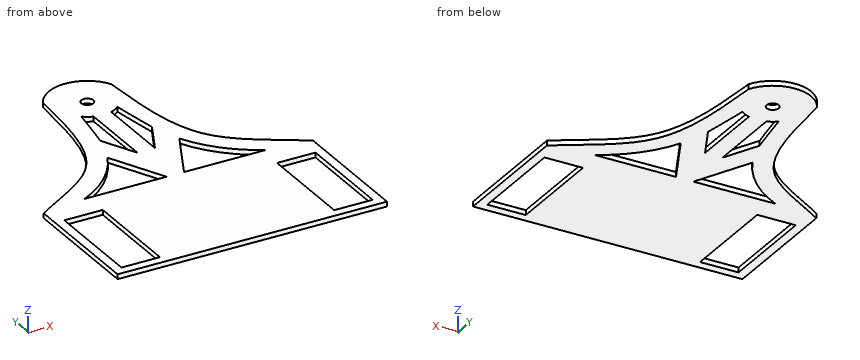
```python
from build123d import *

# Parameters (mm, degrees)
F0_R     = 4
F0_W     = 177.8
F0_H     = 85.24
F0_W_2   = 25.4
F0_H_2   = 66.04
F1_DEPTH = 3.175


with BuildPart() as f1:
    # F0 (on Top) → F1 (new body)
    with BuildSketch(Plane.XY):
        with BuildLine():
            add(Edge.make_bspline(
                [(22.5202294805, 113.3473088044), (24.6785630933, 84.2312430336), (27.5522275569, 27.268327843), (69.7704020362, 9.5247320193), (88.8999999985, -3.66)],
                knots=[0, 0, 0, 0, 0.529467504, 1, 1, 1, 1], degree=3))
            ThreePointArc((22.5202294805, 113.3473088043), (1e-10, 127), (-22.5202294805, 113.3473088044))
            add(Edge.make_bspline(
                [(-22.5202294805, 113.3473088044), (-24.6785630933, 84.2312430336), (-27.5522275569, 27.268327843), (-69.7704020362, 9.5247320193), (-88.8999999985, -3.66)],
                knots=[0, 0, 0, 0, 0.529467504, 1, 1, 1, 1], degree=3))
            Line((-88.8999999985, -3.66), (88.9000000015, -3.66))
        make_face()
        with BuildLine():
            ThreePointArc((-59.8212145269, 0), (-38.7136496278, 15.4052324982), (-23.6512337148, 36.7587828155))
            Line((-23.6512337148, 36.7587828155), (-5.7622946509, 0))
            Line((-5.7622946509, 0), (-59.8212145269, 0))
        make_face(mode=Mode.SUBTRACT)
        with BuildLine():
            Line((5.7622946509, 0), (23.6512337148, 36.7587828155))
            ThreePointArc((23.6512337148, 36.7587828155), (38.7136496278, 15.4052324982), (59.8212145269, 0))
            Line((59.8212145269, 0), (5.7622946509, 0))
        make_face(mode=Mode.SUBTRACT)
        with BuildLine():
            Line((-5.7622946509, 33.5634882355), (-17.0102279312, 56.676113031))
            ThreePointArc((-17.0102279312, 56.676113031), (-14.345117084, 72.11901875), (-11.9453535958, 87.6053768783))
            ThreePointArc((-11.9453535958, 87.6053768783), (-9.0231108807, 85.5649004094), (-5.7622946509, 84.1261077832))
            Line((-5.7622946509, 84.1261077832), (-5.7622946509, 33.5634882355))
        make_face(mode=Mode.SUBTRACT)
        with Locations((0, 101.6)):
            Circle(F0_R, mode=Mode.SUBTRACT)
        with BuildLine():
            Line((5.7622946509, 33.5634882355), (5.7622946509, 84.1261077832))
            ThreePointArc((5.7622946509, 84.1261077832), (9.0231108807, 85.5649004094), (11.9453535958, 87.6053768783))
            ThreePointArc((11.9453535958, 87.6053768783), (14.345117084, 72.11901875), (17.0102279312, 56.676113031))
            Line((17.0102279312, 56.676113031), (5.7622946509, 33.5634882355))
        make_face(mode=Mode.SUBTRACT)
        with Locations((1.5e-09, -46.28)):
            Rectangle(F0_W, F0_H)
        with Locations((-70.1999999985, -49.88)):
            Rectangle(F0_W_2, F0_H_2, mode=Mode.SUBTRACT)
        with Locations((70.1999999985, -49.88)):
            Rectangle(F0_W_2, F0_H_2, mode=Mode.SUBTRACT)
    extrude(amount=F1_DEPTH)


solid = f1.part
```
Source: CAD feature listing. Evaluate the final solid. Frame: model axes, mm. Coordinates: 2 decimals unless noted, no trailing zeros. Write each loop counter-clockwise with the first axis right and the second up, starting at its lowest first coordinate (ties: lowest second). Pieces come first, ordered by that corner, then holes. Notation, with made-up numbers: M 19,61 L 36,61 A33 ccw 36,97 Z; hole C -9,6.5 d3. An arc over 180 degrees is marked long. Answer as a JSON object with one key per item and string values.
1. Contact query for flat-ended pins moving along their axis: P1, Ø1, axis at x = -41.5, z = 2.5, coming from the +Y side; P2, Ø6.5, axis at x = 0, y = 101.6, coming from the -Z side; P3, Ø1, axis at x = 68.5, z = 2.5, coming from the +Y side. Output: stop coordinate, or through.
Evaluation:
{"P1": "y = 31.74", "P2": "through", "P3": "y = 9.58"}
2. Cut plane D-D on x = 20. Output: boundary loops of the cut face in (y, z) (3 decimals).
Evaluation:
{"outline": "M -88.9,0 L 0,0 L 0,3.175 L -88.9,3.175 Z; M 29.256,0 L 117.258,0 L 117.258,3.175 L 29.256,3.175 Z"}
3. Cut plane B-B on z = 2. State how many separate pieces and enclosed holes the cut face has, plus the area to 3 significant figures.
Evaluation:
{"separate pieces": "1", "enclosed holes": "7", "area": "18,700 mm^2"}
4. Ray query, L1, parallel to Y at x = 0, z = 2.45; L2, parallel to Y at x = 58, z = 2.6; L3, parallel to X at y = -60, z = 2.25. Return the intervals inside material, ascending.
Evaluation:
{"L1": "-88.9 to 97.6, 105.6 to 127", "L2": "-88.9 to -82.9, -16.86 to 0, 0.95 to 16.12", "L3": "-88.9 to -82.9, -57.5 to 57.5, 82.9 to 88.9"}
5. Cut plane A-A on x = 0. Output: boundary loops of the cut face in (y, z) (3 decimals), plus the area to 3 significant figures.
Evaluation:
{"outline": "M -88.9,0 L 97.6,0 L 97.6,3.175 L -88.9,3.175 Z; M 105.6,0 L 127,0 L 127,3.175 L 105.6,3.175 Z", "area": "660 mm^2"}
